```python
from build123d import *

# Parameters (mm, degrees)
SKETCH_1_R          = 8
EXTRUDE_1_DEPTH     = 160
SKETCH_2_R          = 4
CUT_EXTRUDE_1_DEPTH = 10
SKETCH_3_R          = 2.5
CUT_EXTRUDE_2_DEPTH = 10


with BuildPart() as part:
    # 草图1 → 凸台-拉伸1 (new body)
    with BuildSketch(Plane.XY):
        Circle(SKETCH_1_R)
    extrude(amount=EXTRUDE_1_DEPTH)

    # 草图2 → 切除-拉伸1 (cut, symmetric)
    with BuildSketch(Plane(origin=(0, 0, 0), x_dir=(1, 0, 0), z_dir=(0, 1, 0))):
        with Locations((0, -150)):
            Circle(SKETCH_2_R)
    extrude(amount=CUT_EXTRUDE_1_DEPTH, both=True, mode=Mode.SUBTRACT)

    # 草图3 → 切除-拉伸2 (cut)
    with BuildSketch(Plane(origin=(0, 0, 0), x_dir=(0, 0, -1), z_dir=(1, 0, 0))):
        with Locations((-4, 0)):
            Circle(SKETCH_3_R)
    extrude(amount=CUT_EXTRUDE_2_DEPTH, mode=Mode.SUBTRACT)


solid = part.part
```
The model under review builds one solid part; all positions refer to its coordinate system, in mm. A direction names the side the tool comes from. Coordinates: 2 decimals unless noted, no trailing zeros. Order: outer loops, then holes, each group sorted by start corner. A loop starts at its lowest first (then second) coordinate and runs counter-clockwise, first axis right, second up. Notation, with made-up numbers: (13.25, 41.5) -> (69.25, 41.5) arc R27 ccw to (69.25, 80.5) -> close; hole circle Ø9 at (13.25, -8). An arc over 180 degrees is marked (long way). Answer in a Markdown table with one row per item. Add a question column.
Item 1: We need section C-C on z = 150. Write out the cut boundary in (x, y), plus the area to 3 significant figures.
Item 2: We need section A-A on y = 0. Write out the cut boundary in (x, z).
Item 3: Clearance check with flat-ended pins moving along their axes: pin 1 (1.5 mm diameter, centred on x = 6, z = 18.5, fed in from -Y); pin 2 (1 mm diameter, centred on x = 5, z = 35.5, fed in from -Y); pin 3 (1.5 mm diameter, centred on y = -3.5, z = 75.5, fed in from +X). State where each tip first meets the part, or that it passes through.
Item 4: Machinability: for faces 5 (the flat face through (0, 0, 4)), 6 (the cylindrical face through (-1.041, 7.932, 78.88)), which of the approach directions +Z, -Z, +X, -X, +Y, -Y give a long, thin tool a straight path to every point of the face, cutting with its end or side? Answer none if there is none.
Item 5: We need section B-B on x = 2. Write out the cut boundary in (y, z).
Item 6: We need section D-D on z = 57. Write out the cut boundary in (x, y).
Item 7: Mouldability with a two-part tool opening along Z and no side actions: class faces 1 (the cylindrical face through (3.944, 0.751, 1.615)), 2 (the flat face through (0, 0, 0)), 3 (the flat face through (0, 0, 160)), 4 (the cylindrical face through (3.815, 0.112, 148.799)) as +Z half, -Z half, draft (parallel to the pull), parting line (faces both ways), or undercut.
Item 8: To check wall thickness, follow probe 1 along Z at (x, y) = (4.75, 0); probe 2 along Z at (x, y) = (2, 0); probe 3 along Z at (x, y) = (0, 3). State the ranges of each line that lie inside material, in increasing order.
Final values:
| question | item | result |
|---|---|---|
| 1 | outline | (-4, -6.93) -> (-4, 6.93) arc R8 ccw to start; (4, -6.93) arc R8 ccw to (4, 6.93) -> close |
| 1 | area | 78.6 mm2 |
| 2 | outline | (-8, 0) -> (8, 0) -> (8, 1.5) -> (0, 1.5) -> (0, 6.5) -> (8, 6.5) -> (8, 160) -> (-8, 160) -> close; hole circle Ø8 at (0, 150) |
| 3 | pin 1 | stops at y = -6.04 |
| 3 | pin 2 | stops at y = -6.61 |
| 3 | pin 3 | stops at x = 7.51 |
| 4 | face 5 | +X |
| 4 | face 6 | +Z, -Z |
| 5 | outline | (-7.75, 0) -> (7.75, 0) -> (7.75, 146.54) -> (-7.75, 146.54) -> close; (-7.75, 153.46) -> (7.75, 153.46) -> (7.75, 160) -> (-7.75, 160) -> close; hole circle Ø5 at (0, 4) |
| 6 | outline | circle Ø16 at (0, 0) |
| 7 | face 1 | undercut |
| 7 | face 2 | -Z half |
| 7 | face 3 | +Z half |
| 7 | face 4 | undercut |
| 8 | probe 1 | z = 0 to 1.5, 6.5 to 160 |
| 8 | probe 2 | z = 0 to 1.5, 6.5 to 146.54, 153.46 to 160 |
| 8 | probe 3 | z = 0 to 146, 154 to 160 |
